from build123d import *

# Parameters (mm, degrees)
SKETCH2_R           = 73.66
SKETCH2_R_2         = 63.5
SKETCH2_R_3         = 1.75
SKETCH2_R_4         = 2.5
BOSS_EXTRUDE1_DEPTH = 5.4356


with BuildPart() as part:
    # Sketch2 → Boss-Extrude1 (new body)
    with BuildSketch(Plane.XY.offset(-69.215)):
        Circle(SKETCH2_R)
        Circle(SKETCH2_R_2, mode=Mode.SUBTRACT)
        with Locations((-68.58, 0)):
            Circle(SKETCH2_R_3, mode=Mode.SUBTRACT)
        with Locations((0, 68.58)):
            Circle(SKETCH2_R_3, mode=Mode.SUBTRACT)
        with Locations((68.58, 0)):
            Circle(SKETCH2_R_3, mode=Mode.SUBTRACT)
        with Locations((0, -68.58)):
            Circle(SKETCH2_R_3, mode=Mode.SUBTRACT)
        with Locations((-24.449968278, 64.073515989)):
            Circle(SKETCH2_R_4, mode=Mode.SUBTRACT)
        with Locations((24.449968278, 64.073515989)):
            Circle(SKETCH2_R_4, mode=Mode.SUBTRACT)
        with Locations((-67.176013668, -13.80578095)):
            Circle(SKETCH2_R_4, mode=Mode.SUBTRACT)
        with Locations((-40.902096909, -55.047569142)):
            Circle(SKETCH2_R_4, mode=Mode.SUBTRACT)
        with Locations((40.902096909, -55.047569142)):
            Circle(SKETCH2_R_4, mode=Mode.SUBTRACT)
        with Locations((67.176013668, -13.80578095)):
            Circle(SKETCH2_R_4, mode=Mode.SUBTRACT)
    extrude(amount=BOSS_EXTRUDE1_DEPTH)


solid = part.part
Model file for the job. Use its own axes, mm. Give positions to 0.01 mm unless a question says otherwise; leave off trailing zeros. Order: outer loops, then holes, each group sorted by start corner. A loop starts at its lowest first (then second) coordinate and runs counter-clockwise, first axis right, second up. Notation, with made-up numbers: (59.25, 78) - (78.25, 78) arc R22 ccw to (78.25, 109) - close; hole circle Ø11 at (68.25, 3.5). An arc over 180 degrees is marked (long way). Write item = value, one per line. Start each with the question number.
1. Probe line 1 along Y through (x, z) = (-39, -64.5); line 2 along Y through (x, z) = (-25, -66.7); line 3 along Y through (x, z) = (46, -65.5) (3 decimals). List the from-to ranges inside material, lowest first.
2. Cut at D-D, the plane z = -66.9. State how many separate pieces and enclosed holes the cut face has, and give its area (3 significant figures).
3. Cut at B-B, the plane x = 17. List the corners of the cut face in (y, z) (3 decimals), and give its area (3 significant figures).
4. Cut at A-A, the plane y = 0. List the corners of the cut face in (x, z) (3 decimals).
5. Cut at C-C, the plane y = -68.58. List the corners of the cut face in (x, z) (3 decimals), and give its area (3 significant figures).
6. Drop flat-ended pins along their axis: P1, Ø1.5, axis at x = -7.5, z = -65.5, coming from the +Y side; P2, Ø1, axis at y = -10.5, z = -64.5, coming from the -X side. Give the stop position or say it passes through.
7. Two-plate mould, pull along X, no slides. Class faces 1 (the flat face through (21.5, 60.4, -63.779)), 2 (the cylindrical face through (-24.78, 66.55, -66.54)), 3 (the cylindrical face through (-58.454, -44.821, -66.535)), 4 (the cylindrical face through (-64.791, -13.055, -66.535)): pulls with the +X half, pulls with the -X half, needs draft (parallel to the pull), parting line crosses it, or undercut.
Taken from the geometry:
q1.line_1 = -62.49 to -56.67, -53.43 to -50.11, 50.11 to 62.49
q1.line_2 = -69.29 to -58.37, 58.37 to 61.63, 66.51 to 69.29
q1.line_3 = -57.531 to -43.775, 43.775 to 57.531
q2.separate_pieces = 1
q2.enclosed_holes = 11
q2.area = 4,220 mm²
q3.outline = (-71.671, -69.215) - (-61.182, -69.215) - (-61.182, -63.779) - (-71.671, -63.779) - close; (61.182, -69.215) - (71.671, -69.215) - (71.671, -63.779) - (61.182, -63.779) - close
q3.area = 114 mm²
q4.outline = (-73.66, -69.215) - (-70.33, -69.215) - (-70.33, -63.779) - (-73.66, -63.779) - close; (-66.83, -69.215) - (-63.5, -69.215) - (-63.5, -63.779) - (-66.83, -63.779) - close; (63.5, -69.215) - (66.83, -69.215) - (66.83, -63.779) - (63.5, -63.779) - close; (70.33, -69.215) - (73.66, -69.215) - (73.66, -63.779) - (70.33, -63.779) - close
q5.outline = (-26.881, -69.215) - (-1.75, -69.215) - (-1.75, -63.779) - (-26.881, -63.779) - close; (1.75, -69.215) - (26.881, -69.215) - (26.881, -63.779) - (1.75, -63.779) - close
q5.area = 273 mm²
q6.P1 = 73.35
q6.P2 = -72.98
q7.face_1 = needs draft
q7.face_2 = undercut
q7.face_3 = parting line crosses it
q7.face_4 = undercut
